from build123d import *

# Parameters (mm, degrees)
F0_W     = 1.1
F0_H     = 0.4
F1_DEPTH = 0.7
F2_R     = 0.1
F4_DEPTH = 25
F5_SCALE = 15


with BuildPart() as f1:
    # F0 (on Front) → F1 (new body)
    with BuildSketch(Plane.XZ):
        with Locations((0, 0.2)):
            Rectangle(F0_W, F0_H)
        Polygon((0.55, 0), (-0.55, 0), (-0.8, 0), (-0.8, -0.2), (0.8, -0.2), (0.8, 0), align=None)
    extrude(amount=F1_DEPTH)

    # F2
    f2_edges = [f1.edges().sort_by_distance(p)[0] for p in [
        (-0.55, -0.35, 0.4),
        (0.55, -0.35, 0.4),
    ]]
    fillet(f2_edges, radius=F2_R)

    # F3 (on face) → F4 (cut)
    with BuildSketch(Plane.XY):
        with BuildLine():
            Line((-0.8, -0.25), (-0.8, -0.45))
            ThreePointArc((-0.8, -0.45), (-0.7, -0.35), (-0.8, -0.25))
        make_face()
        with BuildLine():
            Line((0.8, -0.45), (0.8, -0.25))
            ThreePointArc((0.8, -0.25), (0.7, -0.35), (0.8, -0.45))
        make_face()
    extrude(amount=-F4_DEPTH, mode=Mode.SUBTRACT)


with BuildPart() as f1_1:
    # F5: moved
    add(f1.part.scale(F5_SCALE))


solid = f1_1.part
For this review, take the finished solid that the model builds, in its own axes (mm). A direction names the side the tool comes from. Coordinates: 2 decimals unless noted, no trailing zeros. Order: outer loops, then holes, each group sorted by start corner. A loop starts at its lowest first (then second) coordinate and runs counter-clockwise, first axis right, second up. Notation, with made-up numbers: (-18.75, 69) - (26.25, 69) arc R31 ccw to (26.25, 106) - close; hole circle Ø11 at (-24.5, -39). An arc over 180 degrees is marked (long way). Use one line per item in the form item = value.
Q1. For faces 1 (the flat face through (8.25, -5, 2)), 2 (the cylindrical face through (10.5, -5.2, -1.5)), 3 (the flat face through (-8.25, -5, 2)), list the 3-axis set-ups (+Z, -Z, +X, -X, +Y, -Y) from which the entire face can be reached by the end or side of a thin tool; tool diameter is ignored.
Checked values:
face_1 = +Z, +X, +Y, -Y
face_2 = +Z, -Z, +X
face_3 = +Z, -X, +Y, -Y
Q2. For probe 1 along Z at (x, y) = (9.5, -3); probe 2 along X at (y, z) = (-2.5, 2.5); probe 3 along Z at (x, y) = (7.5, -2.25), list the stretches that pass through material, from the lowest coordinate up. Write a range as from..to.
Checked values:
probe_1 = -3..0
probe_2 = -8.25..8.25
probe_3 = -3..5.8
Q3. Draft analysis for pull direction Y (two halves, no side actions). For faces 4 (the flat face through (10, -5, 0)), 5 (the cylindrical face through (-10.5, -5.3, -1.5)), 6 (the flat face through (0, 0, 2)), 7 (the flat face through (0, -10.5, 2)), state which applies: +Y half, -Y half, draft (parallel to the pull), parting line (faces both ways), or undercut.
Checked values:
face_4 = draft
face_5 = undercut
face_6 = +Y half
face_7 = -Y half
Q4. Consider section D-D (z = 0.5). Give the boundary of the cut face in (x, y), then the cut area to 3 significant figures.
Checked values:
outline = (-8.25, -10.5) - (8.25, -10.5) - (8.25, 0) - (-8.25, 0) - close
area = 173 mm2
Q5. Consider section A-A (z = -0.5). Give the boundary of the cut face in (x, y), then the cut area to 3 significant figures.
Checked values:
outline = (-12, -10.5) - (12, -10.5) - (12, -6.75) arc R1.5 cw to (12, -3.75) - (12, 0) - (-12, 0) - (-12, -3.75) arc R1.5 cw to (-12, -6.75) - close
area = 245 mm2
Q6. Consider section C-C (y = -7.75). Give the boundary of the cut face in (x, z), then the cut area to 3 significant figures.
Checked values:
outline = (-12, -3) - (12, -3) - (12, 0) - (8.25, 0) - (8.25, 4.5) arc R1.5 ccw to (6.75, 6) - (-6.75, 6) arc R1.5 ccw to (-8.25, 4.5) - (-8.25, 0) - (-12, 0) - close
area = 170 mm2
Q7. For P1, Ø1.1, axis at x = -10, y = -5, coming from the +Z side; P2, Ø3, axis at y = -7.5, z = 4.5, coming from the +X side; P3, Ø2.5, axis at y = -4.5, z = 3, coming from the -X side, all flat-tipped, find the tip position at first contact; note any pin that passes through.
Checked values:
P1 = 0
P2 = 8.25
P3 = -8.25
Q8. Consider section B-B (y = -5.25). Give the boundary of the cut face in (x, z), then the cut area to 3 significant figures.
Checked values:
outline = (-10.5, -3) - (10.5, -3) - (10.5, 0) - (8.25, 0) - (8.25, 4.5) arc R1.5 ccw to (6.75, 6) - (-6.75, 6) arc R1.5 ccw to (-8.25, 4.5) - (-8.25, 0) - (-10.5, 0) - close
area = 161 mm2
